```python
from build123d import *

# Parameters (mm, degrees)
SKETCH_1_W        = 30
SKETCH_1_H        = 120
EXTRUDE_1_DEPTH   = 2
CHAMFER_1_SIZE    = 2
HOLE_WIZARD_M61_D = 6.6


with BuildPart() as part:
    # Эскиз1 → Бобышка-Вытянуть1 (new body)
    with BuildSketch(Plane.XY):
        Rectangle(SKETCH_1_W, SKETCH_1_H)
    extrude(amount=EXTRUDE_1_DEPTH)

    # Фаска1
    chamfer_1_edges = [part.edges().sort_by_distance(p)[0] for p in [
        (15, -60, 1),
        (-15, -60, 1),
        (-15, 60, 1),
        (15, 60, 1),
    ]]
    chamfer(chamfer_1_edges, length=CHAMFER_1_SIZE)

    # Отверстие с зазором M61 (through all)
    with Locations(Plane.XY.offset(2)):
        with Locations((0, -45), (0, 45), (0, 15), (0, -15)):
            Hole(HOLE_WIZARD_M61_D / 2)


solid = part.part
```
The model under review builds one solid part; all positions refer to its coordinate system, in mm. Coordinates: 2 decimals unless noted, no trailing zeros. Write each loop counter-clockwise with the first axis right and the second up, starting at its lowest first coordinate (ties: lowest second). Pieces come first, ordered by that corner, then holes. Notation, with made-up numbers: (7.25, 65) -> (52.25, 65) arc R30 cw to (52.25, 96) -> close; hole circle Ø4 at (65.25, -22.5). An arc over 180 degrees is marked (long way). One line per item, written item: value. Start each with the question number.
Q1. To check wall thickness, follow probe 1 along Y at (x, z) = (0, 1.1); probe 2 along Y at (x, z) = (-1.25, 0.55); probe 3 along X at (y, z) = (46, 0.2). State the ranges of each line that lie inside material, in increasing order.
Q2. Add section C-C, the plane z = 0.5. Give the boundary of the cut face in (x, y).
Q3. Add section B-B, the plane y = 15. Give the boundary of the cut face in (x, z).
Q4. The part is to be moulded in two halves that separate along Y. For faces 1 (the face through (-15, -1, 1)), 2 (the face through (0, 60, 1)), 3 (the face through (0, -60, 1)), 4 (the face through (0.43, -41.73, 0.99)), say which applies: +Y half, -Y half, draft (parallel to the pull), parting line (faces both ways), or undercut.
Q5. Clearance check with flat-ended pins moving along their axes: P1, Ø4, axis at x = 0, y = -45, coming from the +Z side; P2, Ø7.5, axis at x = 0, y = 45, coming from the +Z side. State where each tip first meets the part, or that it passes through.
Q6. Add section A-A, the plane x = 0. Give the boundary of the cut face in (y, z), then the cut area to 3 significant figures.
Response:
1. probe 1: -60 to -48.3, -41.7 to -18.3, -11.7 to 11.7, 18.3 to 41.7, 48.3 to 60
1. probe 2: -60 to -48.05, -41.95 to -18.05, -11.95 to 11.95, 18.05 to 41.95, 48.05 to 60
1. probe 3: -15 to -3.14, 3.14 to 15
2. outline: (-15, -58) -> (-13, -60) -> (13, -60) -> (15, -58) -> (15, 58) -> (13, 60) -> (-13, 60) -> (-15, 58) -> close; hole circle Ø6.6 at (0, -45); hole circle Ø6.6 at (0, -15); hole circle Ø6.6 at (0, 15); hole circle Ø6.6 at (0, 45)
3. outline: (-15, 0) -> (-3.3, 0) -> (-3.3, 2) -> (-15, 2) -> close; (3.3, 0) -> (15, 0) -> (15, 2) -> (3.3, 2) -> close
4. face 1: draft
4. face 2: +Y half
4. face 3: -Y half
4. face 4: undercut
5. P1: through
5. P2: z = 2
6. outline: (-60, 0) -> (-48.3, 0) -> (-48.3, 2) -> (-60, 2) -> close; (-41.7, 0) -> (-18.3, 0) -> (-18.3, 2) -> (-41.7, 2) -> close; (-11.7, 0) -> (11.7, 0) -> (11.7, 2) -> (-11.7, 2) -> close; (18.3, 0) -> (41.7, 0) -> (41.7, 2) -> (18.3, 2) -> close; (48.3, 0) -> (60, 0) -> (60, 2) -> (48.3, 2) -> close
6. area: 187 mm²
